Autodesk Inventor part; units mm, degrees
ref_plane "YZ Plane" through (0, 0, 0) normal (1, 0, 0) x (0, 1, 0)
ref_plane "XZ Plane" through (0, 0, 0) normal (0, 1, 0) x (-1, 0, 0)
ref_plane "XY Plane" through (0, 0, 0) normal (0, 0, 1) x (1, 0, 0)
sketch "Sketch1" plane through (0, 0, 0) normal (0, 1, 0) x (-1, 0, 0)
  line L0 (0, 22.5) -> (-17.6777, 40.1777)
  line L1 (0, -22.5) -> (-17.6777, -40.1777)
  line L2 (0, 0) -> (0, 13)
  line L3 (0, 13) -> (0, -13)
  line L4 (-17.6777, 40.1777) -> (-19.799, 38.0563)
  line L5 (0, 22.5) -> (-2.1213, 20.3787)
  line L6 (-2.1213, 20.3787) -> (-19.799, 38.0563)
  line L7 (-2.1213, -20.3787) -> (-19.799, -38.0563)
  line L8 (-19.799, -38.0563) -> (-17.6777, -40.1777)
  line L9 (-2.1213, -20.3787) -> (0, -22.5)
  circle A0 centre (0, -17.5) radius 1.525
  circle A1 centre (0, 17.5) radius 1.525
  line L10 (0, -22.5) -> (2, -20.5)
  line L11 (0, -13) -> (2, -15)
  line L12 (0, 22.5) -> (2, 20.5)
  line L13 (0, 13) -> (2, 15)
  line L14 (0, -22.5) -> (-18.3848, -40.8848)
  line L15 (-18.3848, -40.8848) -> (-20.5061, -38.7635)
  line L16 (-20.5061, -38.7635) -> (-19.799, -38.0563)
  line L17 (-19.799, 38.0563) -> (-20.5061, 38.7635)
  line L18 (-20.5061, 38.7635) -> (-18.3848, 40.8848)
  line L19 (-18.3848, 40.8848) -> (-17.6777, 40.1777)
  line L20 (0, -13) -> (-2.1213, -15)
  line L21 (-2.1213, -20.3787) -> (-4.8107, -17.6893)
  line L22 (-2.1213, -20.3787) -> (1.682, -20.3787) construction
  line L23 (-4.8107, -17.6893) -> (-2.1213, -15)
  line L24 (2, -20.5) -> (4.75, -17.75)
  line L25 (4.75, -17.75) -> (2, -15)
  line L26 (0, 13) -> (-2.1213, 15.1213)
  line L27 (-2.1213, 15.1213) -> (-4.75, 17.75)
  line L28 (-4.75, 17.75) -> (-2.1213, 20.3787)
  line L29 (2, 15) -> (4.75, 17.75)
  line L30 (4.75, 17.75) -> (2, 20.5)
  line L31 (-2.1213, -15) -> (-2.1213, 15.1213)
  dimension "d3" = 25
  dimension "d6" = 25
  dimension "d8" = 13
  dimension "d9" = 26
  dimension "d10" = 3
  dimension "d12" = 3.05
  dimension "d13" = 3.05
  dimension "d16" = 26
  dimension "d17" = 135
extrude "Extrusion2" add sketch "Sketch1" along normal blind 8
sketch "Sketch3" plane through (0, 0, -13) normal (-1, 0, 0) x (0, 0, 1)
  point P0 (13, 0)
sketch "Sketch4" plane through (0, 0, -13) normal (-1, 0, 0) x (0, 0, 1)
  line L0 (13, 0) -> (13, 5)
  line L1 (13, 5) -> (3, 5)
  line L2 (3, 5) -> (23, 5)
  circle A0 centre (3, 5) radius 1.55
  circle A1 centre (23, 5) radius 1.55
  dimension "d20" = 5
  dimension "d21" = 10
  dimension "d22" = 20
  dimension "d23" = 3.1
  dimension "d24" = 3.1
extrude "Extrusion3" cut sketch "Sketch4" against normal blind 8
sketch "Sketch5" plane through (-4.75, 0, -17.75) normal (-0.7071, 0, -0.7071) x (-0.7071, 0, 0.7071)
  line L0 (-6.7175, 0) -> (-32.7175, 0)
  line L1 (-32.7175, 0) -> (-6.7175, 0)
  line L2 (-19.7175, 0) -> (-19.7175, 5)
  line L3 (-19.7175, 5) -> (-29.7175, 5)
  line L4 (-29.7175, 5) -> (-9.7175, 5)
  circle A0 centre (-29.7175, 5) radius 1.55
  circle A1 centre (-9.7175, 5) radius 1.55
  point P0 (9.1924, 0)
  dimension "d27" = 5
  dimension "d28" = 10
  dimension "d29" = 20
  dimension "d30" = 3.1
  dimension "d31" = 3.1
extrude "Extrusion4" cut sketch "Sketch5" against normal blind 8
sketch "Sketch6" plane through (18.3848, 0, 40.8848) normal (-0.7071, 0, 0.7071) x (0.7071, 0, 0.7071)
  line L0 (-32.7175, 0) -> (0, 0)
  line L1 (0, 0) -> (-26, 0)
  line L2 (0, 0) -> (-13, 0)
  line L3 (-13, 0) -> (-13, 5)
  line L4 (-13, 5) -> (-23, 5)
  line L5 (-23, 5) -> (-3, 5)
  circle A0 centre (-23, 5) radius 1.55
  circle A1 centre (-3, 5) radius 1.55
  point P0 (-41.9099, 0)
  dimension "d34" = 26
  dimension "d35" = 13
  dimension "d36" = 5
  dimension "d37" = 10
  dimension "d38" = 20
  dimension "d39" = 3.1
  dimension "d40" = 3.1
extrude "Extrusion5" cut sketch "Sketch6" against normal blind 8
properties part number "distanceSensorMount"
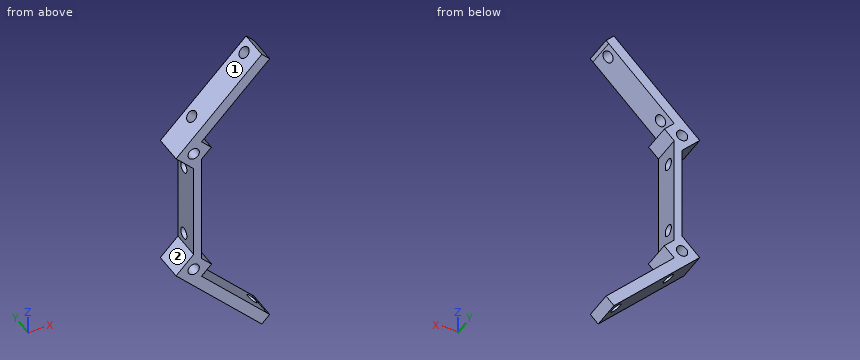
Can you work these out from the model? Positions are in its coordinate system, mm. Face numbers are marked on the shaded views. Coordinates: 2 decimals unless noted, no trailing zeros. Order: outer loops, then holes, each group sorted by start corner. A loop starts at its lowest first (then second) coordinate and runs counter-clockwise, first axis right, second up. Notation, with made-up numbers: (56, 45) - (109, 45) arc R13 ccw to (109, 62) - close; hole circle Ø4 at (39.5, 3). An arc over 180 degrees is marked (long way). Answer in a Markdown table with one row per item.
1. If we mould it in two halves opening along Z, with no side actions, what happens to the marked faces 1 and 2? For each: pulls with the +Z half, pulls with the -Z half, needs draft (parallel to the pull), parting line crosses it, or undercut.
Reply:
| item | result |
|---|---|
| face 1 | pulls with the +Z half |
| face 2 | undercut |
2. Suppose I cut it at B-B (x = 11.75). Please give me the cut outline in (y, z).
Reply:
| item | result |
|---|---|
| outline | (0, -34.25) - (8, -34.25) - (8, -30.01) - (0, -30.01) - close; (0, 30.01) - (8, 30.01) - (8, 34.25) - (0, 34.25) - close |
3. For pin 1 (5 mm diameter, centred on x = 0, z = 17.5, fed in from +Y); pin 2 (3 mm diameter, centred on x = 9.5, y = 3.5, fed in from -Z); pin 3 (4 mm diameter, centred on x = 12, y = 1.5, fed in from -Z); pin 4 (2.5 mm diameter, centred on y = 2.5, z = 4, fed in from +X), each with a flat end and sliding along its axis, tell me the tip position at first contact or that it passes through.
Reply:
| item | result |
|---|---|
| pin 1 | stops at y = 8 |
| pin 2 | stops at z = -33.5 |
| pin 3 | stops at z = -36.5 |
| pin 4 | stops at x = 2.12 |
4. If I drill on line 1 along Y through (x, z) = (0.8, -10); line 2 along Z through (x, y) = (1.25, 1.5); line 3 along Z through (x, y) = (-0.75, 6.5), over which ranges is the centre line in solid material (lowest first)?
Reply:
| item | result |
|---|---|
| line 1 | y = 0 to 3.45, 6.55 to 8 |
| line 2 | z = -23.75 to -18.37, -16.63 to 16.63, 18.37 to 23.75 |
| line 3 | z = -21.75 to -18.83, -16.17 to -13.75, 13.75 to 16.17, 18.83 to 21.75 |
5. Suppose I cut it at A-A (z = -10). Please give me the cut outline in (x, y), and give its area (3 significant figures).
Reply:
| item | result |
|---|---|
| outline | (0, 0) - (2.12, 0) - (2.12, 3.45) - (0, 3.45) - close; (0, 6.55) - (2.12, 6.55) - (2.12, 8) - (0, 8) - close |
| area | 10.4 mm^2 |
6. Suppose I cut it at D-D (z = 27). Please give me the cut outline in (x, y), and give its area (3 significant figures).
Reply:
| item | result |
|---|---|
| outline | (4.5, 0) - (8.74, 0) - (8.74, 8) - (4.5, 8) - close |
| area | 33.9 mm^2 |
7. Suppose I cut it at C-C (y = 2.75). Give the number of separate pieces and of enclosed holes in the cut face, and give its area (3 significant figures).
Reply:
| item | result |
|---|---|
| separate pieces | 1 |
| enclosed holes | 2 |
| area | 292 mm^2 |
